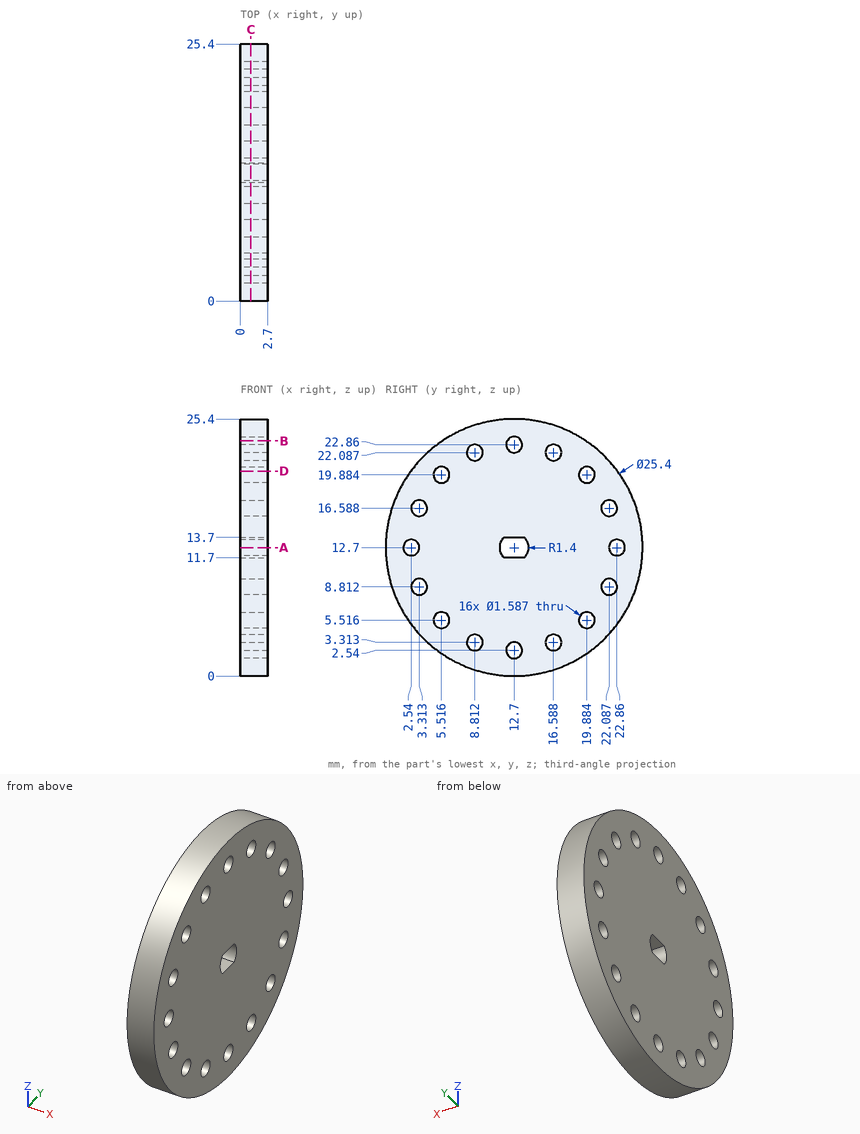
Input: dimensioned drawing with shaded views. Units: mm. Origin: part minimum x, y, z. Give positions to 0.01 mm unless a question says otherwise; leave off trailing zeros. Order: outer loops, then holes, each group sorted by start corner. A loop starts at its lowest first (then second) coordinate and runs counter-clockwise, first axis right, second up.
(1) Section query B-B (z = 23.25). Return the cut outline in (x, y).
(2) Section query D-D (z = 20.25). Return the cut outline in (x, y).
(3) Material intervals for line 1 along Z through (x, y) = (1.65, 9.5) (1 decimal); line 2 along Z through (x, y) = (2.15, 19.5) (1 decimal); line 3 along Y through (x, z) = (0.95, 20.5) (1 decimal), sorted ascending.
(4) Contact query for a flat-ended pin moving along its axis: P1, Ø1.5, axis at x = 1, y = 9, coming from the -Z side. Output: stop coordinate, or through.
(5) Section query C-C (x = 1.05). State how many separate pieces and enclosed holes the cut face has, plus the area to 3 significant figures.
(6) Section query A-A (z = 12.7). Return the cut outline in (x, y).
Outcome:
1. outline: (0, 5.63) - (2.7, 5.63) - (2.7, 12.01) - (0, 12.01) - close; (0, 13.39) - (2.7, 13.39) - (2.7, 19.77) - (0, 19.77) - close
2. outline: (0, 2.49) - (2.7, 2.49) - (2.7, 4.81) - (0, 4.81) - close; (0, 6.22) - (2.7, 6.22) - (2.7, 19.18) - (0, 19.18) - close; (0, 20.59) - (2.7, 20.59) - (2.7, 22.91) - (0, 22.91) - close
3. line 1: z = 0.4 to 2.9, 3.7 to 21.7, 22.5 to 25
3. line 2: z = 2 to 4.8, 6.2 to 19.2, 20.6 to 23.4
3. line 3: y = 2.7 to 5, 6 to 19.4, 20.4 to 22.7
4. P1: stops at z = 0.35
5. separate pieces: 1
5. enclosed holes: 17
5. area: 470 mm2
6. outline: (0, 0) - (2.7, 0) - (2.7, 1.75) - (0, 1.75) - close; (0, 3.33) - (2.7, 3.33) - (2.7, 11.3) - (0, 11.3) - close; (0, 14.1) - (2.7, 14.1) - (2.7, 22.07) - (0, 22.07) - close; (0, 23.65) - (2.7, 23.65) - (2.7, 25.4) - (0, 25.4) - close
